Geometry check sheet. Reference: the model listing, model coordinates, mm. A direction names the side the tool comes from. Round coordinates to 2 decimals unless told otherwise and drop trailing zeros. Order: outer loops, then holes, each group sorted by start corner. A loop starts at its lowest first (then second) coordinate and runs counter-clockwise, first axis right, second up. Notation, with made-up numbers: (-24, 32) - (32, 32) arc R28 cw to (32, 56) - close; hole circle Ø1 at (62, 17.25). An arc over 180 degrees is marked (long way). Return JSON: item names as keys, results as strings. Group by question number.
Q1. Sectioned sample at B-B, the plane z = 32.5. Record the cut outline in (x, y), then the cut area to 3 significant figures.
Q2. Sectioned sample at A-A, the plane y = 27. Record the cut outline in (x, z), then the cut area to 3 significant figures.
Q3. Tool access check on faces 3 (the flat face through (-59.47, 15, 21)), 4 (the flat face through (-74, 1.5, 33)), 5 (the flat face through (-56.8, 38.5, 44.2)), 6 (the cylindrical face through (-60.896, 0.76, 26.088)), 7 (the flat face through (-76, 16, 24.584)). Record the directions out of +Z, -Z, +X, -X, +Y, -Y that give a thin tool (end or side, any length) a straight path to the whole face; none if there is none.
Q4. Sectioned sample at C-C, the plane x = -63. Record the cut outline in (y, z).
Q5. Material ranges on line 1 along X through (y, z) = (4.5, 41.25); line 2 along X through (y, z) = (12.5, 44.5); line 3 along Z through (x, y) = (-58.5, 5), recorded low to high.
Q6. Gauge pin test, flat ends, axial feed: pin 1 Ø5 at (x, z) = (-70, 37) entering from +Y; pin 2 Ø0.8 at (x, z) = (-75.5, 32) entering from +Y; pin 3 Ø1.2 at (x, y) = (-76, 25.5) entering from -Z. Record the tip position at first contact, or that the pin passes through.
Q7. Draft check along Z on faces 1 (the flat face through (-73, 19, 43.984)), 2 (the cylindrical face through (-61.181, 6.304, 20.845)). Enter one of: pulls with the +Z half, pulls with the -Z half, needs draft (parallel to the pull), parting line crosses it, or undercut.
Q8. Sectioned sample at D-D, the plane y = 18. Record the cut outline in (x, z), then the cut area to 3 significant figures.
```python
from build123d import *

# Parameters (mm, degrees)
SKETCH1_W           = 21.6
SKETCH1_H           = 25.4
BOSS_EXTRUDE1_DEPTH = 38.5
SKETCH2_W           = 18.6
SKETCH2_H           = 22.4
CUT_EXTRUDE1_DEPTH  = 37
CUT_EXTRUDE2_DEPTH  = 25.5
CUT_EXTRUDE3_DEPTH  = 25.5
CUT_EXTRUDE4_DEPTH  = 1.5
FILLET2_R           = 3
FILLET3_R           = 3
SKETCH7_W           = 21.6
SKETCH7_H           = 4.5
CUT_EXTRUDE5_DEPTH  = 18.5


with BuildPart() as part:
    # Sketch1 → Boss-Extrude1 (new body)
    with BuildSketch(Plane(origin=(0, 0, 0), x_dir=(1, 0, 0), z_dir=(0, 1, 0))):
        with Locations((-65.770128024, -32.78448737)):
            Rectangle(SKETCH1_W, SKETCH1_H)
    extrude(amount=BOSS_EXTRUDE1_DEPTH)

    # Sketch2 → Cut-Extrude1 (cut)
    with BuildSketch(Plane(origin=(0, 38.5, 0), x_dir=(1, 0, 0), z_dir=(0, 1, 0))):
        with Locations((-65.770128024, -32.78448737)):
            Rectangle(SKETCH2_W, SKETCH2_H)
    extrude(amount=-CUT_EXTRUDE1_DEPTH, mode=Mode.SUBTRACT)

    # Sketch5 → Cut-Extrude2 (cut)
    with BuildSketch(Plane.XY.offset(45.48448737)):
        with BuildLine():
            Line((-72.070128024, 38.5), (-59.470128024, 38.5))
            Line((-59.470128024, 38.5), (-59.470128024, 10.5))
            ThreePointArc((-59.470128024, 10.5), (-61.227487337, 6.257359313), (-65.470128024, 4.5))
            Line((-65.470128024, 4.5), (-66.070128024, 4.5))
            ThreePointArc((-66.070128024, 4.5), (-70.312768711, 6.257359313), (-72.070128024, 10.5))
            Line((-72.070128024, 10.5), (-72.070128024, 38.5))
        make_face()
    extrude(amount=-CUT_EXTRUDE2_DEPTH, mode=Mode.SUBTRACT)

    # Sketch3 → Cut-Extrude3 (cut)
    with BuildSketch(Plane(origin=(-54.970128024, 0, 0), x_dir=(0, 0, -1), z_dir=(1, 0, 0))):
        with BuildLine():
            Line((-40.98448737, 38.5), (-24.58448737, 38.5))
            Line((-24.58448737, 38.5), (-24.58448737, 11))
            ThreePointArc((-24.58448737, 11), (-26.488293292, 6.403805922), (-31.08448737, 4.5))
            Line((-31.08448737, 4.5), (-34.48448737, 4.5))
            ThreePointArc((-34.48448737, 4.5), (-39.080681448, 6.403805922), (-40.98448737, 11))
            Line((-40.98448737, 11), (-40.98448737, 38.5))
        make_face()
    extrude(amount=-CUT_EXTRUDE3_DEPTH, mode=Mode.SUBTRACT)

    # Sketch6 → Cut-Extrude4 (cut)
    with BuildSketch(Plane(origin=(0, 1.5, 0), x_dir=(1, 0, 0), z_dir=(0, 1, 0))):
        with BuildLine():
            Line((-67.070128024, -40.98448737), (-64.470128024, -40.98448737))
            ThreePointArc((-64.470128024, -40.98448737), (-60.934594118, -39.520021276), (-59.470128024, -35.98448737))
            Line((-59.470128024, -35.98448737), (-59.470128024, -29.58448737))
            ThreePointArc((-59.470128024, -29.58448737), (-60.934594118, -26.048953464), (-64.470128024, -24.58448737))
            Line((-64.470128024, -24.58448737), (-67.070128024, -24.58448737))
            ThreePointArc((-67.070128024, -24.58448737), (-70.60566193, -26.048953464), (-72.070128024, -29.58448737))
            Line((-72.070128024, -29.58448737), (-72.070128024, -35.98448737))
            ThreePointArc((-72.070128024, -35.98448737), (-70.60566193, -39.520021276), (-67.070128024, -40.98448737))
        make_face()
    extrude(amount=-CUT_EXTRUDE4_DEPTH, mode=Mode.SUBTRACT)

    # Fillet2
    fillet2_edges = [part.edges().sort_by_distance(p)[0] for p in [
        (-65.770128024, 1.5, 43.98448737),
    ]]
    fillet(fillet2_edges, radius=FILLET2_R - 0.0001)  # a hair under: the kernel refuses the full size

    # Fillet3
    fillet3_edges = [part.edges().sort_by_distance(p)[0] for p in [
        (-65.770128024, 1.5, 21.58448737),
    ]]
    fillet(fillet3_edges, radius=FILLET3_R - 0.0001)  # a hair under: the kernel refuses the full size

    # Sketch7 → Cut-Extrude5 (cut)
    with BuildSketch(Plane(origin=(0, 38.5, 0), x_dir=(1, 0, 0), z_dir=(0, 1, 0))):
        with Locations((-65.770128024, -22.33448737)):
            Rectangle(SKETCH7_W, SKETCH7_H)
    extrude(amount=-CUT_EXTRUDE5_DEPTH, mode=Mode.SUBTRACT)


solid = part.part
```
Reply:
{
 "1": {"outline": "(-76.57, 0) - (-72.07, 0) - (-72.07, 1.5) - (-75.07, 1.5) - (-75.07, 4.5) - (-76.57, 4.5) - close; (-59.47, 0) - (-54.97, 0) - (-54.97, 4.5) - (-56.47, 4.5) - (-56.47, 1.5) - (-59.47, 1.5) - close", "area": "22.5 mm^2"},
 "2": {"outline": "(-76.57, 40.98) - (-75.07, 40.98) - (-75.07, 43.98) - (-72.07, 43.98) - (-72.07, 45.48) - (-76.57, 45.48) - close; (-59.47, 43.98) - (-56.47, 43.98) - (-56.47, 40.98) - (-54.97, 40.98) - (-54.97, 45.48) - (-59.47, 45.48) - close", "area": "22.5 mm^2"},
 "3": {"face 3": "+Z, -Z, +Y", "face 4": "+Y", "face 5": "+Z, -Z, +X, -X, +Y", "face 6": "+Y, -Y", "face 7": "+X, -X, +Y"},
 "4": {"outline": "(0, 20.08) - (5.03, 20.08) - (5.03, 21.58) - (4.5, 21.58) arc R3 cw to (1.5, 24.58) - (1.5, 24.81) - (0, 24.81) - close; (0, 40.76) - (1.5, 40.76) - (1.5, 40.98) arc R3 cw to (4.5, 43.98) - (5.03, 43.98) - (5.03, 45.48) - (0, 45.48) - close"},
 "5": {"line 1": "-76.57 to -75.07, -56.47 to -54.97", "line 2": "-76.57 to -72.07, -59.47 to -54.97", "line 3": "20.08 to 21.58, 43.98 to 45.48"},
 "6": {"pin 1": "y = 1.5", "pin 2": "y = 4.5", "pin 3": "z = 40.98"},
 "7": {"face 1": "undercut", "face 2": "needs draft"},
 "8": {"outline": "(-76.57, 20.08) - (-72.07, 20.08) - (-72.07, 21.58) - (-75.07, 21.58) - (-75.07, 24.58) - (-76.57, 24.58) - close; (-76.57, 40.98) - (-75.07, 40.98) - (-75.07, 43.98) - (-72.07, 43.98) - (-72.07, 45.48) - (-76.57, 45.48) - close; (-59.47, 20.08) - (-54.97, 20.08) - (-54.97, 24.58) - (-56.47, 24.58) - (-56.47, 21.58) - (-59.47, 21.58) - close; (-59.47, 43.98) - (-56.47, 43.98) - (-56.47, 40.98) - (-54.97, 40.98) - (-54.97, 45.48) - (-59.47, 45.48) - close", "area": "45.0 mm^2"}
}
